The listing builds one solid part. Answer for the finished solid, in the listing's coordinates (mm). Round coordinates to 2 decimals unless told otherwise and drop trailing zeros. Order: outer loops, then holes, each group sorted by start corner. A loop starts at its lowest first (then second) coordinate and runs counter-clockwise, first axis right, second up. Notation, with made-up numbers: M 87,-33 L 109,-33 A13 ccw 109,-14 Z; hole C 50.5,56.25 d7. An arc over 180 degrees is marked long. Write item = value, one per line. Start each with the question number.
(1) Straight lines are drawn through the part: probe 1 along Z at (x, y) = (6.5, 1.45); probe 2 along X at (y, z) = (1.9, 10.5); probe 3 along X at (y, z) = (2.75, 9.25). For each, find the intervals that lie inside material, in ascending order. Write a range as from..to.
(2) A cutting plane is placed at A-A, the plane z = 10.5. Determine the outline of the cut face in (x, y).
(3) Each of these flat-tipped pins is pushed along its axis until it touches: pin 1 (1 mm diameter, centred on y = 3.5, z = 8.5, fed in from -X); pin 2 (1.3 mm diameter, centred on y = 1.5, z = 2.5, fed in from +X); pin 3 (4 mm diameter, centred on x = 6.5, z = 3.5, fed in from +Y); pin 4 (2.5 mm diameter, centred on x = 6.5, z = 10.5, fed in from -Y). Where does it stop, or does it pass through?
(4) A cutting plane is placed at B-B, the plane x = 117. Determine the outline of the cut face in (y, z).
Autodesk Inventor part; units mm, degrees
ref_plane "YZ Plane" through (0, 0, 0) normal (1, 0, 0) x (0, 1, 0)
ref_plane "XZ Plane" through (0, 0, 0) normal (0, 1, 0) x (-1, 0, 0)
ref_plane "XY Plane" through (0, 0, 0) normal (0, 0, 1) x (1, 0, 0)
sketch "Sketch1" plane through (0, 0, 0) normal (0, 0, 1) x (1, 0, 0)
  line L0 (0, 0) -> (0, 2.5)
  line L1 (2, 4.5) -> (11, 4.5)
  line L2 (0, 2.5) -> (2, 4.5)
  line L3 (0, 8.8411) -> (0, 0) construction
  line L4 (43, 7) -> (92.5, 7)
  line L5 (43, 11.0001) -> (43, -2.4525) construction
  line L6 (43, 7) -> (11, 4.5)
  line L7 (92.5, 7) -> (124.5, 4.5)
  line L8 (0, 0) -> (149.0621, 0)
  line L9 (124.5, 4.5) -> (124.5, 0)
  dimension "d0" = 4.5
  dimension "d1" = 45
  dimension "d2" = 7
  dimension "d3" = 9
  dimension "d4" = 32
  dimension "d5" = 49.5
  dimension "d8" = 32
  dimension "d9" = 2
  dimension "d10" = 4.5
extrude "Extrusion1" add sketch "Sketch1" along normal blind 14
sketch "Sketch2" plane through (124.5, 0, 0) normal (1, 0, 0) x (0, 0, -1)
  circle A0 centre (-7, 2.25) radius 2.25
  line L0 (0, 4.5) -> (-14, 4.5)
  line L1 (-7, 4.5) -> (-7, -0.9771) construction
  line L2 (0, 2.5) -> (-14, 2.5)
  point P0 (0, 0)
  dimension "d13" = 4.5
extrude "Extrusion2" add sketch "Sketch2" along normal blind 4.5
sketch "Sketch3" plane through (2, 4.5, 0) normal (0, 1, 0) x (1, 0, 0)
  circle A0 centre (4.5, -3.5) radius 1.5
  circle A1 centre (4.5, -10.5) radius 1.5
  line L0 (9, 0) -> (0, 0)
  line L1 (9, -14) -> (0, -14)
  line L2 (0, 0) -> (0, -14)
  point P0 (-2, 0)
  dimension "d16" = 7
  dimension "d17" = 3.5
  dimension "d18" = 3.5
  dimension "d19" = 4.5
  dimension "d20" = 3
  dimension "d21" = 3
extrude "Extrusion3" cut sketch "Sketch3" against normal blind 4.5
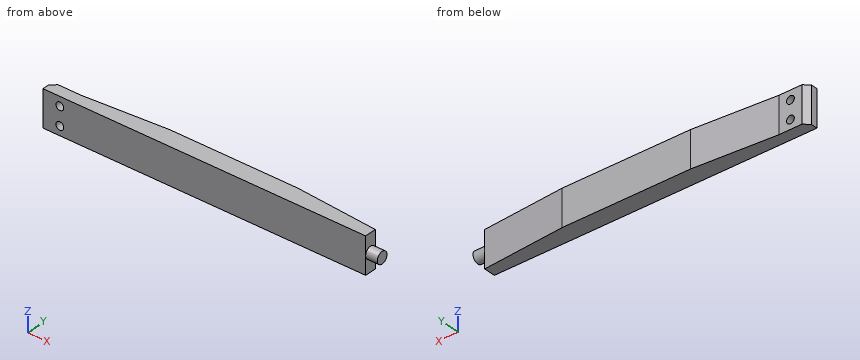
Reported:
q1.probe_1 = 0..2, 5..9, 12..14
q1.probe_2 = 0..5, 8..124.5
q1.probe_3 = 0.25..5.67, 7.33..124.5
q2.outline = M 0,0 L 5,0 L 5,4.5 L 2,4.5 L 0,2.5 Z; M 8,0 L 124.5,0 L 124.5,4.5 L 92.5,7 L 43,7 L 11,4.5 L 8,4.5 Z
q3.pin_1 = 0.5
q3.pin_2 = 124.5
q3.pin_3 = 4.5
q3.pin_4 = through
q4.outline = M 0,0 L 5.09,0 L 5.09,14 L 0,14 Z
